Read the model definition and answer for the solid it produces. Units are mm, in the model's axes. Coordinates: 2 decimals unless noted, no trailing zeros. Write each loop counter-clockwise with the first axis right and the second up, starting at its lowest first coordinate (ties: lowest second). Pieces come first, ordered by that corner, then holes.
(1) Straight lines are drawn through the part: line 1 along Y through (x, z) = (80, 3.75); line 2 along Y through (x, z) = (30, 5.5); line 3 along X through (y, z) = (91, 6.25). For each, find the intervals that lie inside material, in ascending order.
(2) The part is cut by section C-C, the plane z = 6.75. State how many separate pieces and enclosed holes the cut face has, and give its area (3 significant figures).
(3) The part is cut by section A-A, the plane y = 30. Determine the outline of the cut face in (x, z), and give its area (3 significant figures).
```python
from build123d import *

# Parameters (mm, degrees)
SKETCH_1_W      = 200
SKETCH_1_H      = 200
SKETCH_1_R      = 3.25
SKETCH_1_R_2    = 4.25
EXTRUDE_1_DEPTH = 10
FILLET_1_R      = 20


with BuildPart() as part:
    # 草图1 → 凸台-拉伸1 (new body)
    with BuildSketch(Plane.XY):
        Rectangle(SKETCH_1_W, SKETCH_1_H)
        with Locations((30, 30)):
            Circle(SKETCH_1_R, mode=Mode.SUBTRACT)
        with Locations(Location((30, -30, 0), (0, 0, 180))):
            Circle(SKETCH_1_R, mode=Mode.SUBTRACT)
        with Locations(Location((-30, 30, 0), (0, 0, 180))):
            Circle(SKETCH_1_R, mode=Mode.SUBTRACT)
        with Locations((-30, -30)):
            Circle(SKETCH_1_R, mode=Mode.SUBTRACT)
        with Locations((80, 80)):
            Circle(SKETCH_1_R_2, mode=Mode.SUBTRACT)
        with Locations(Location((80, -80, 0), (0, 0, 180))):
            Circle(SKETCH_1_R_2, mode=Mode.SUBTRACT)
        with Locations((-80, -80)):
            Circle(SKETCH_1_R_2, mode=Mode.SUBTRACT)
        with Locations(Location((-80, 80, 0), (0, 0, 180))):
            Circle(SKETCH_1_R_2, mode=Mode.SUBTRACT)
    extrude(amount=EXTRUDE_1_DEPTH)

    # 圆角1
    fillet_1_edges = [part.edges().sort_by_distance(p)[0] for p in [
        (-100, 100, 5),
        (-100, -100, 5),
        (100, -100, 5),
        (100, 100, 5),
    ]]
    fillet(fillet_1_edges, radius=FILLET_1_R)


solid = part.part
```
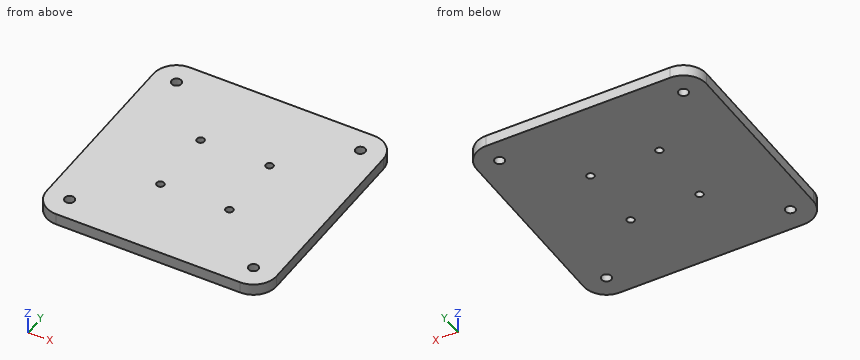
Computed:
1. line 1: y = -100 to -84.25, -75.75 to 75.75, 84.25 to 100
1. line 2: y = -100 to -33.25, -26.75 to 26.75, 33.25 to 100
1. line 3: x = -96.7 to 96.7
2. separate pieces: 1
2. enclosed holes: 8
2. area: 39,300 mm2
3. outline: (-100, 0) - (-33.25, 0) - (-33.25, 10) - (-100, 10) - close; (-26.75, 0) - (26.75, 0) - (26.75, 10) - (-26.75, 10) - close; (33.25, 0) - (100, 0) - (100, 10) - (33.25, 10) - close
3. area: 1,870 mm2
